Read the model definition and answer for the solid it produces. Units are mm, in the model's axes. Coordinates: 2 decimals unless noted, no trailing zeros. Loops run counter-clockwise (first coordinate to the right, second up) from the corner with the lowest first, then second, coordinate; pieces in that order, holes last. Notation, with made-up numbers: (56.25, 20.25) -> (60.25, 20.25) arc R24 ccw to (60.25, 55.25) -> close; hole circle Ø4 at (66.5, -31). An arc over 180 degrees is marked (long way). Answer in a Markdown table with one row per item.
```python
from build123d import *

# Parameters (mm, degrees)
F0_W     = 176.5
F0_H     = 115
F0_W_2   = 5
F0_H_2   = 5
F1_DEPTH = 2


with BuildPart() as f1:
    # F0 (on Top) → F1 (new body)
    with BuildSketch(Plane.XY):
        Polygon((-88.25, 62.5), (-88.25, 57.5), (-93.25, 57.5), (-93.25, -62.5), (93.25, -62.5), (93.25, 62.5), align=None)
        Rectangle(F0_W, F0_H, mode=Mode.SUBTRACT)
        with Locations((-90.75, 60)):
            Rectangle(F0_W_2, F0_H_2)
    extrude(amount=F1_DEPTH)


solid = f1.part
```
1. Find the intervals of material crossed by probe 1 along Y at (x, z) = (-50.5, 1.05); probe 2 along X at (y, z) = (49, 0.7), in increasing order.
A:
| item | result |
|---|---|
| probe 1 | y = -62.5 to -57.5, 57.5 to 62.5 |
| probe 2 | x = -93.25 to -88.25, 88.25 to 93.25 |
2. A cutting plane is placed at B-B on z = 1.55. Give the vertices of the cut face in (x, y), and give its area (4 significant figures).
A:
| item | result |
|---|---|
| outline | (-93.25, -62.5) -> (93.25, -62.5) -> (93.25, 62.5) -> (-93.25, 62.5) -> close; hole (-88.25, -57.5) -> (88.25, -57.5) -> (88.25, 57.5) -> (-88.25, 57.5) -> close |
| area | 3,015 mm2 |
3. A cutting plane is placed at A-A on y = -42.5. Give the vertices of the cut face in (x, z), and give its area (3 significant figures).
A:
| item | result |
|---|---|
| outline | (-93.25, 0) -> (-88.25, 0) -> (-88.25, 2) -> (-93.25, 2) -> close; (88.25, 0) -> (93.25, 0) -> (93.25, 2) -> (88.25, 2) -> close |
| area | 20.0 mm2 |
4. A cutting plane is placed at C-C on x = -80.5. Give the vertices of the cut face in (y, z).
A:
| item | result |
|---|---|
| outline | (-62.5, 0) -> (-57.5, 0) -> (-57.5, 2) -> (-62.5, 2) -> close; (57.5, 0) -> (62.5, 0) -> (62.5, 2) -> (57.5, 2) -> close |
